Model file for the job. Use its own axes, mm. A direction names the side the tool comes from. Round coordinates to 2 decimals unless told otherwise and drop trailing zeros. Loops run counter-clockwise (first coordinate to the right, second up) from the corner with the lowest first, then second, coordinate; pieces in that order, holes last. Notation, with made-up numbers: (52, 1.5) -> (107, 1.5) arc R27 ccw to (107, 22.5) -> close; hole circle Ø11 at (45.25, 53.5). An arc over 180 degrees is marked (long way). Use a Markdown table: item, result.
from build123d import *

# Parameters (mm, degrees)
F0_R     = 2.38125
F1_DEPTH = 50.76
F2_R     = 3


with BuildPart() as f1:
    # F0 (on Front) → F1 (new body)
    with BuildSketch(Plane.XZ):
        Polygon((13.911133, -49.24), (30, -49.24), (30, -44.24), (13.911133, -44.24), (13.911133, -31.161906), (38.442495, -16.998718), (33.442495, -8.338464), (0, -27.646497), (-33.442495, -8.338464), (-38.442495, -16.998718), (-13.911133, -31.161906), (-13.911133, -44.24), (-30, -44.24), (-30, -49.24), (-13.911133, -49.24), align=None)
        with Locations((-28.942569, -16.71)):
            Circle(F0_R, mode=Mode.SUBTRACT)
        with Locations((28.942569, -16.71)):
            Circle(F0_R, mode=Mode.SUBTRACT)
    extrude(amount=F1_DEPTH)

    # F2
    f2_edges = [f1.edges().sort_by_distance(p)[0] for p in [
        (-33.442495, -25.38, -8.338464),
        (-38.442495, -25.38, -16.998718),
        (0, -25.38, -27.646497),
        (33.442495, -25.38, -8.338464),
        (38.442495, -25.38, -16.998718),
        (13.911133, -25.38, -31.161906),
        (13.911133, -25.38, -44.24),
        (-13.911133, -25.38, -31.161906),
        (-13.911133, -25.38, -44.24),
        (-30, -25.38, -44.24),
        (30, -25.38, -44.24),
    ]]
    fillet(f2_edges, radius=F2_R)


solid = f1.part
Q1. Band-saw the part on B-B, the plane z = -16.71. Give the cut face in (x, y).
Results list:
| item | result |
|---|---|
| outline | (-37.23, -50.76) -> (-31.32, -50.76) -> (-31.32, 0) -> (-37.23, 0) -> close; (-26.56, -50.76) -> (-18.94, -50.76) -> (-18.94, 0) -> (-26.56, 0) -> close; (18.94, -50.76) -> (26.56, -50.76) -> (26.56, 0) -> (18.94, 0) -> close; (31.32, -50.76) -> (37.23, -50.76) -> (37.23, 0) -> (31.32, 0) -> close |
Q2. Tool access for faces 5 (the face through (30, -25, -48)), 6 (the face through (-22, -25, -44.24)), 7 (the face through (29.1, -25.7, -45.1)): list every direction of +Z, -Z, +X, -X, +Y, -Y with a clear straight run to the whole face (end or side of a thin tool).
Results list:
| item | result |
|---|---|
| face 5 | -Z, +X, +Y, -Y |
| face 6 | -X, +Y, -Y |
| face 7 | +X, +Y, -Y |
Q3. Flat gauge pins, fed straight in: pin 1 (6 mm diameter, centred on x = -8.5, y = -37.5, fed in from +Z); pin 2 (3 mm diameter, centred on x = 23, y = -20, fed in from +Z); pin 3 (6 mm diameter, centred on y = -23, z = -24, fed in from -X); pin 4 (3 mm diameter, centred on x = -28.94, z = -16.71, fed in from +Y). Where does each tip first touch, or does it go through?
Results list:
| item | result |
|---|---|
| pin 1 | stops at z = -21.01 |
| pin 2 | stops at z = -13.5 |
| pin 3 | stops at x = -31.51 |
| pin 4 | passes through |
Q4. Band-saw the part on C-C, the plane x = 24. Give the cut face in (y, z).
Results list:
| item | result |
|---|---|
| outline | (-50.76, -49.24) -> (0, -49.24) -> (0, -44.24) -> (-50.76, -44.24) -> close; (-50.76, -25.34) -> (0, -25.34) -> (0, -13.79) -> (-50.76, -13.79) -> close |
Q5. Drill centre lines: L1, parallel to Z at x = -27.5, y = -30.5; L2, parallel to Z at x = -29.5, y = -23.5; L3, parallel to X at y = -31, z = -17. Where is each one in solid material? Low to high. Write a range as from..to.
Results list:
| item | result |
|---|---|
| L1 | z = -49.24..-44.28, -23.32..-18.6, -14.82..-11.77 |
| L2 | z = -49.24..-45.58, -22.16..-19.03, -14.39..-10.61 |
| L3 | x = -37.14..-31.31, -26.58..-18.44, 18.44..26.58, 31.31..37.14 |
Q6. Band-saw the part on D-D, the plane z = -21. Give the cut face in (x, y).
Results list:
| item | result |
|---|---|
| outline | (-31.51, -50.76) -> (-11.51, -50.76) -> (-11.51, 0) -> (-31.51, 0) -> close; (11.51, -50.76) -> (31.51, -50.76) -> (31.51, 0) -> (11.51, 0) -> close |
Q7. Pull direction X, two halves, no side cores. Call faces 1 (the face through (35.956, -25.025, -12.693)), 2 (the face through (-14.81, -25.74, -43.38)), 3 (the face through (-33.153, -25.735, -9.547)), 4 (the face through (26.564, -25.025, -16.605)): released by +X, released by -X, zero draft, split by the parting line, or undercut.
Results list:
| item | result |
|---|---|
| face 1 | released by +X |
| face 2 | released by -X |
| face 3 | undercut |
| face 4 | undercut |
Q8. Band-saw the part on A-A, the plane y = -37.5. Give the cut face in (x, z).
Results list:
| item | result |
|---|---|
| outline | (-36.94, -14.4) arc R3 ccw to (-35.84, -18.5) -> (-15.41, -30.3) arc R3 cw to (-13.91, -32.89) -> (-13.91, -41.24) arc R3 cw to (-16.91, -44.24) -> (-27, -44.24) arc R3 ccw to (-30, -47.24) -> (-30, -49.24) -> (30, -49.24) -> (30, -47.24) arc R3 ccw to (27, -44.24) -> (16.91, -44.24) arc R3 cw to (13.91, -41.24) -> (13.91, -32.89) arc R3 cw to (15.41, -30.3) -> (35.84, -18.5) arc R3 ccw to (36.94, -14.4) -> (34.94, -10.94) arc R3 ccw to (30.84, -9.84) -> (1.5, -26.78) arc R3 cw to (-1.5, -26.78) -> (-30.84, -9.84) arc R3 ccw to (-34.94, -10.94) -> close; hole circle Ø4.76 at (-28.94, -16.71); hole circle Ø4.76 at (28.94, -16.71) |
